For this review, take the finished solid that the model builds, in its own axes (mm). A direction names the side the tool comes from. Give positions to 0.01 mm unless a question says otherwise; leave off trailing zeros. Order: outer loops, then holes, each group sorted by start corner. A loop starts at its lowest first (then second) coordinate and runs counter-clockwise, first axis right, second up. Notation, with made-up numbers: M -15,57.25 L -7,57.25 A37 cw -7,94.25 Z; hole C -37,-9.75 d8. An arc over 180 degrees is marked long. Use CSV: the item, a comma, the result in double quotes. Start each with the question number.
(1) Wall thickness on L1, parallel to Y at x = 0, z = 1.75; L2, parallel to X at y = -3, z = 8.5; L3, parallel to Y at x = 0, z = 10.25: over which ranges is each line inside the solid? List them lowest first. Write a range as from..to.
(2) Clearance check with flat-ended pins moving along their axes: P1, Ø1.6, axis at x = -14.5, y = -1, coming from the -Z side; P2, Ø3, axis at x = 11.5, y = 4, coming from the -Z side; P3, Ø4.5, axis at x = 1, y = 3, coming from the +Z side; P4, Ø3, axis at x = 1.5, y = -2, coming from the +Z side. State where each tip first meets the part, or that it passes through.
(3) Draft analysis for pull direction Y (two halves, no side actions). For faces 1 (the face through (-5, 2.65, 16)), 2 (the face through (-0.596, 0.315, 9.969)), 3 (the face through (0, -6.35, 7)), state which applies: pulls with the +Y half, pulls with the -Y half, needs draft (parallel to the pull), parting line crosses it, or undercut.
(4) Consider section C-C (z = 10.75). Write out the cut boundary in (x, y).
(5) Consider section D-D (x = -3.5). Write out the cut boundary in (y, z), and give its area (3 significant figures).
(6) Consider section A-A (y = 4). Write out the cut boundary in (x, z).
(7) Consider section B-B (x = 1). Write out the cut boundary in (y, z).
(8) Tool access review of faces 4 (the face through (-5, -3.35, 16)), 5 (the face through (-11, 0, 19.5)), 6 (the face through (14.36, 2.39, 1.97)), 7 (the face through (0, -5, 7)), 8 (the face through (0, 6, 12)): name each direction out of +Z, -Z, +X, -X, +Y, -Y from which nothing blocks a thin tool from reaching the whole face with its end or side.
```python
from build123d import *

# Parameters (mm, degrees)
SKETCH2_W           = 32
SKETCH2_H           = 12.7
SKETCH2_R           = 1.75
BOSS_EXTRUDE1_DEPTH = 19.5
SKETCH3_R           = 1.75
CUT_EXTRUDE1_DEPTH  = 20.5
CUT_EXTRUDE2_DEPTH  = 4
SKETCH5_R           = 8
CUT_EXTRUDE3_DEPTH  = 3.7
SKETCH9_R           = 6
CUT_EXTRUDE5_DEPTH  = 6
SKETCH10_R          = 8
CUT_EXTRUDE6_DEPTH  = 4
SKETCH6_R           = 2.75
CUT_EXTRUDE4_DEPTH  = 7.5


with BuildPart() as part:
    # Sketch2 → Boss-Extrude1 (new body)
    with BuildSketch(Plane.XY):
        Rectangle(SKETCH2_W, SKETCH2_H)
        with Locations((0, 3)):
            Circle(SKETCH2_R, mode=Mode.SUBTRACT)
        with Locations((0, -3)):
            Circle(SKETCH2_R, mode=Mode.SUBTRACT)
    extrude(amount=BOSS_EXTRUDE1_DEPTH)

    # Sketch3 → Cut-Extrude1 (cut, through all)
    with BuildSketch(Plane.XY.offset(19.5)):
        with Locations((-13, 0)):
            Circle(SKETCH3_R)
        with Locations((13, 0)):
            Circle(SKETCH3_R)
    extrude(amount=-CUT_EXTRUDE1_DEPTH, mode=Mode.SUBTRACT)

    # Sketch4 → Cut-Extrude2 (cut)
    with BuildSketch(Plane(origin=(0, 0, 0), x_dir=(-1, 0, 0), z_dir=(0, 0, -1))):
        Polygon((-10.25, -1.58771324), (-10.25, 1.58771324), (-13, 3.175426481), (-15.75, 1.58771324), (-15.75, -1.58771324), (-13, -3.175426481), align=None)
        Polygon((13, -3.175426481), (15.75, -1.58771324), (15.75, 1.58771324), (13, 3.175426481), (10.25, 1.58771324), (10.25, -1.58771324), align=None)
    extrude(amount=-CUT_EXTRUDE2_DEPTH, mode=Mode.SUBTRACT)

    # Sketch5 → Cut-Extrude3 (cut)
    with BuildSketch(Plane(origin=(0, 6.35, 0), x_dir=(1, 0, 0), z_dir=(0, 1, 0))):
        with Locations((0, -20)):
            Circle(SKETCH5_R)
    extrude(amount=-CUT_EXTRUDE3_DEPTH, mode=Mode.SUBTRACT)

    # Sketch9 → Cut-Extrude5 (cut)
    with BuildSketch(Plane(origin=(0, 2.65, 0), x_dir=(1, 0, 0), z_dir=(0, 1, 0))):
        with Locations((0, -20)):
            Circle(SKETCH9_R)
    extrude(amount=-CUT_EXTRUDE5_DEPTH, mode=Mode.SUBTRACT)

    # Sketch10 → Cut-Extrude6 (cut, through all)
    with BuildSketch(Plane(origin=(0, -3.35, 0), x_dir=(1, 0, 0), z_dir=(0, 1, 0))):
        with Locations((0, -20)):
            Circle(SKETCH10_R)
    extrude(amount=-CUT_EXTRUDE6_DEPTH, mode=Mode.SUBTRACT)

    # Sketch6 → Cut-Extrude4 (cut)
    with BuildSketch(Plane.XY.offset(14.5)):
        with Locations((0, 3)):
            Circle(SKETCH6_R)
        with Locations((0, -3)):
            Circle(SKETCH6_R)
    extrude(amount=-CUT_EXTRUDE4_DEPTH, mode=Mode.SUBTRACT)


solid = part.part
```
Check result:
1,L1,"y = -6.35..-4.75, -1.25..1.25, 4.75..6.35"
1,L2,"x = -16..-2.75, 2.75..16"
1,L3,"y = -6.35..-5.75, -0.25..0.25, 5.75..6.35"
2,P1,"stops at z = 4"
2,P2,"stops at z = 0"
2,P3,"stops at z = 14.94"
2,P4,"stops at z = 14.8"
3,face 1,"pulls with the +Y half"
3,face 2,"undercut"
3,face 3,"pulls with the -Y half"
4,outline,"M -16,-6.35 L 16,-6.35 L 16,6.35 L -16,6.35 Z; hole C -13,0 d3.5; hole C 0,-3 d5.5; hole C 0,3 d5.5; hole C 13,0 d3.5"
5,outline,"M -6.35,0 L 6.35,0 L 6.35,12.81 L 2.65,12.81 L 2.65,15.13 L -3.35,15.13 L -3.35,12.81 L -6.35,12.81 Z"
5,area,"177 mm^2"
6,outline,"M -16,0 L -1.44,0 L -1.44,7 L -2.56,7 L -2.56,12.42 A8 cw -7.98,19.5 L -16,19.5 Z; M 1.44,0 L 16,0 L 16,19.5 L 7.98,19.5 A8 cw 2.56,12.42 L 2.56,7 L 1.44,7 Z"
7,outline,"M -6.35,0 L -4.44,0 L -4.44,7 L -5.56,7 L -5.56,12.06 L -6.35,12.06 Z; M -1.56,0 L 1.56,0 L 1.56,7 L 0.44,7 L 0.44,14.08 L -0.44,14.08 L -0.44,7 L -1.56,7 Z; M 4.44,0 L 6.35,0 L 6.35,12.06 L 5.56,12.06 L 5.56,7 L 4.44,7 Z"
8,face 4,"+Z, -Y"
8,face 5,"+Z, +X, -X, +Y, -Y"
8,face 6,"-Z"
8,face 7,"none"
8,face 8,"+Z, +Y"
